CAD build for the part. Positions are in the model's coordinates, mm. Face numbers are marked on the shaded views. A direction names the side the tool comes from. Round coordinates to 2 decimals unless told otherwise and drop trailing zeros. Loops run counter-clockwise (first coordinate to the right, second up) from the corner with the lowest first, then second, coordinate; pieces in that order, holes last.
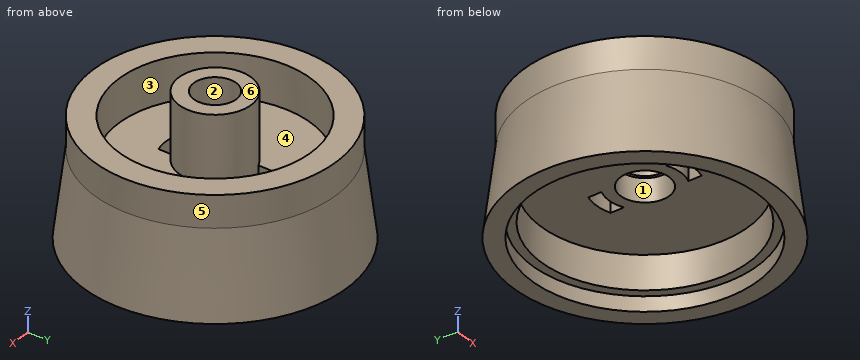
```python
from build123d import *

# Parameters (mm, degrees)
SKETCH_1_R           = 1.7
SKETCH_1_R_2         = 1
EXTRUDE_1_DEPTH      = 1.1
EXTRUDE_1_DEPTH_BACK = 2
SKETCH_1_3_R         = 5.7
SKETCH_1_3_R_2       = 4.525
EXTRUDE_2_DEPTH      = 1.5
SKETCH_2_R           = 5
EXTRUDE_3_DEPTH      = 1.2
SKETCH_2_5_R         = 1
CUT_EXTRUDE_3_DEPTH  = 2.2
SKETCH_6_R           = 1.15
CUT_EXTRUDE_4_DEPTH  = 1.1
SKETCH_4_W           = 0.5
SKETCH_4_H           = 0.375
SKETCH_7_R           = 5.325
CUT_EXTRUDE_5_DEPTH  = 0.7


with BuildPart() as part:
    # Sketch 1 → Extrude 1 (new body, two sides)
    with BuildSketch(Plane.XY) as extrude_1_sk:
        Circle(SKETCH_1_R)
        Circle(SKETCH_1_R_2, mode=Mode.SUBTRACT)
    extrude(amount=EXTRUDE_1_DEPTH)
    extrude(extrude_1_sk.sketch, amount=-EXTRUDE_1_DEPTH_BACK)

    # Sketch 2 → Extrude 3 (add)
    with BuildSketch(Plane(origin=(0, 0, -2), x_dir=(-1, 0, 0), z_dir=(0, 0, -1))):
        Circle(SKETCH_2_R)
    extrude(amount=EXTRUDE_3_DEPTH)

    # Sketch 2_5 → Cut-Extrude 3 (cut, through all)
    with BuildSketch(Plane(origin=(0, 0, -2), x_dir=(-1, 0, 0), z_dir=(0, 0, -1))):
        with BuildLine():
            Line((-0.7, -1.549193338), (-0.7, -2.19089023))
            ThreePointArc((-0.7, -2.19089023), (0, -2.3), (0.7, -2.19089023))
            Line((0.7, -2.19089023), (0.7, -1.549193338))
            ThreePointArc((0.7, -1.549193338), (0, -1.7), (-0.7, -1.549193338))
        make_face()
        with BuildLine():
            ThreePointArc((0.7, 2.19089023), (0, 2.3), (-0.7, 2.19089023))
            Line((-0.7, 2.19089023), (-0.7, 1.549193338))
            ThreePointArc((-0.7, 1.549193338), (0, 1.7), (0.7, 1.549193338))
            Line((0.7, 1.549193338), (0.7, 2.19089023))
        make_face()
        with BuildLine():
            Line((-0.7, -1.549193338), (-0.7, -2.19089023))
            ThreePointArc((-0.7, -2.19089023), (0, -2.3), (0.7, -2.19089023))
            Line((0.7, -2.19089023), (0.7, -1.549193338))
            ThreePointArc((0.7, -1.549193338), (0, -1.7), (-0.7, -1.549193338))
        make_face()
        with BuildLine():
            ThreePointArc((0.7, 2.19089023), (0, 2.3), (-0.7, 2.19089023))
            Line((-0.7, 2.19089023), (-0.7, 1.549193338))
            ThreePointArc((-0.7, 1.549193338), (0, 1.7), (0.7, 1.549193338))
            Line((0.7, 1.549193338), (0.7, 2.19089023))
        make_face()
        with Locations(Location((0, 0, 0), (0, 0, 180))):  # turned: the seam where the file's is
            Circle(SKETCH_2_5_R)
    extrude(amount=CUT_EXTRUDE_3_DEPTH, mode=Mode.SUBTRACT)

    # Sketch 6 → Cut-Extrude 4 (cut)
    with BuildSketch(Plane(origin=(0, 0, -3.2), x_dir=(-1, 0, 0), z_dir=(0, 0, -1))):
        Circle(SKETCH_6_R)
    extrude(amount=-CUT_EXTRUDE_4_DEPTH, mode=Mode.SUBTRACT)



with BuildPart() as body_2:
    # Sketch 1_3 → Extrude 2 (new body)
    with BuildSketch(Plane.XY):
        Circle(SKETCH_1_3_R)
        Circle(SKETCH_1_3_R_2, mode=Mode.SUBTRACT)
    extrude(amount=-EXTRUDE_2_DEPTH)


with BuildPart() as part_1:
    add(part.part)

    add(body_2.part)  # Revolve 2 merges body 2
    # Sketch 4 → Revolve 2 (revolve)
    with BuildSketch(Plane(origin=(0, 0, 0), x_dir=(0, 0, -1), z_dir=(1, 0, 0)), mode=Mode.PRIVATE) as revolve_2_sk:
        Polygon((1.5, 5.7), (5.5, 6.2), (5.5, 4.9), (1.5, 4.9), align=None)
        with Locations((1.75, 4.7125)):
            Rectangle(SKETCH_4_W, SKETCH_4_H)
    revolve(revolve_2_sk.sketch.rotate(Axis((0, 0, 1000), (0, 0, -1)), 90), axis=Axis((0, 0, 1000), (0, 0, -1)))  # turned: the seam where the file's is

    # Sketch 7 → Cut-Extrude 5 (cut)
    with BuildSketch(Plane(origin=(0, 0, -5.5), x_dir=(-1, 0, 0), z_dir=(0, 0, -1))):
        Circle(SKETCH_7_R)
    extrude(amount=-CUT_EXTRUDE_5_DEPTH, mode=Mode.SUBTRACT)


solid = part_1.part
```
Item 1: Cut at A-A, the plane x = 0. State how many separate pieces and enclosed holes the cut face has, plus the area to 3 significant figures.
Answers follow:
separate pieces: 4
enclosed holes: 0
area: 23.6 mm2
Item 2: Two-plate mould, pull along Y, no slides. Class the marked faces 4, 5 and 6: released by +Y, released by -Y, zero draft, split by the parting line, or undercut.
Answers follow:
face 4: undercut
face 5: split by the parting line
face 6: zero draft
Item 3: Flat gauge pins, fed straight in: P1, Ø0.7, axis at y = 2, z = -3, coming from the -X side; P2, Ø1, axis at y = 1, z = -1, coming from the +X side; P3, Ø1.2, axis at x = -0.5, y = -0.5, coming from the -Z side. Where does each tip first touch, or does it go through?
Answers follow:
P1: stops at x = -5.66
P2: stops at x = 5.68
P3: stops at z = -3.2
Item 4: 3-axis set-ups, long thin cutter, end or side, ignore diameter. For the marked faces 1, 2 and 3: which of +Z, -Z, +X, -X, +Y, -Y reach the whole face in a straight line?
Answers follow:
face 1: -Z
face 2: +Z, -Z
face 3: +Z
Item 5: Cut at D-D, the plane z = -4.25. Give the cut face in (x, y), plus the area to 3 significant figures.
Answers follow:
outline: circle Ø12.09 at (0, 0); hole circle Ø9.8 at (0, 0)
area: 39.3 mm2
Item 6: Cut at C-C, the plane z = -0.25. Give the cut face in (x, y) (3 decimals).
Answers follow:
outline: circle Ø11.4 at (0, 0); circle Ø3.4 at (0, 0); hole circle Ø9.05 at (0, 0); hole circle Ø2 at (0, 0)
Item 7: Probe line 1 (Y direction, x = 0, z = -2.6); line 2 (X direction, y = -0.25, z = -0.25); line 3 (Y direction, x = 2, z = -4.75). List the from-to ranges inside material, lowest first.
Answers follow:
line 1: y = -5.84 to -2.3, -1.7 to -1.15, 1.15 to 1.7, 2.3 to 5.84
line 2: x = -5.69 to -4.52, -1.68 to -0.97, 0.97 to 1.68, 4.52 to 5.69
line 3: y = -5.77 to -4.47, 4.47 to 5.77
